from build123d import *

# Parameters (mm, degrees)
EXTRUSION1_DEPTH = 182
CONG_1_R         = 0.5


with BuildPart() as part:
    # Esquisse1 → Extrusion1 (new body)
    with BuildSketch(Plane(origin=(0, 0, 0), x_dir=(1, 0, 0), z_dir=(0, 1, 0))):
        with BuildLine():
            Line((5.5, 0), (-5.5, 0))
            Line((-5.5, 0), (-5.5, 2.476845379))
            ThreePointArc((-5.5, 2.476845379), (-4.1, 4), (-5.5, 5.523154621))
            Line((-5.5, 5.523154621), (-5.5, 6))
            Line((-5.5, 6), (-4.9, 6))
            ThreePointArc((-4.9, 6), (-3.5, 4), (-4.9, 2))
            Line((-4.9, 2), (-4.9, 0.6))
            Line((-4.9, 0.6), (4.9, 0.6))
            Line((4.9, 0.6), (4.9, 2))
            ThreePointArc((4.9, 2), (3.5, 4), (4.9, 6))
            Line((4.9, 6), (5.5, 6))
            Line((5.5, 6), (5.5, 5.523154621))
            ThreePointArc((5.5, 5.523154621), (4.1, 4), (5.5, 2.476845379))
            Line((5.5, 2.476845379), (5.5, 0))
        make_face()
    extrude(amount=EXTRUSION1_DEPTH)

    # Congé1
    cong_1_edges = [part.edges().sort_by_distance(p)[0] for p in [
        (5.5, 91, 0),
        (-5.5, 91, 0),
    ]]
    fillet(cong_1_edges, radius=CONG_1_R)


solid = part.part
Source: CAD feature listing. Evaluate the final solid. Frame: model axes, mm. A direction names the side the tool comes from. Coordinates: 2 decimals unless noted, no trailing zeros. Order: outer loops, then holes, each group sorted by start corner. A loop starts at its lowest first (then second) coordinate and runs counter-clockwise, first axis right, second up. Notation, with made-up numbers: M 37.5,-3 L 58.5,-3 A15 cw 58.5,7 Z; hole C -8.5,22 d2. An arc over 180 degrees is marked long. Write each question's results on one line, items separated by ' | '. Start each with the question number.
1. Section B-B, the plane z = -4.5. Return the cut outline in (x, y), then the cut area to 3 significant figures.
2. Section A-A, the plane y = 146. Return the cut outline in (x, z), then the cut area to 3 significant figures.
3. Pin query (flat end, axial travel): pin 1 (3 mm diameter, centred on x = 4, z = -2.5, fed in from -Y); pin 2 (5 mm diameter, centred on x = 0, y = 125, fed in from -Z). Return the tip coordinate at first contact, or that it passes through.
4. Draft query along Z for faces 3 (the face through (0, 90, 0)), 4 (the face through (0, 90, -0.6)), 5 (the face through (0, 182, -0.3)). Return one class per face: +Z half, -Z half, draft (parallel to the pull), parting line (faces both ways), or undercut.
5. Section C-C, the plane x = 0.75. Return the cut outline in (y, z), then the cut area to 3 significant figures.
6. Material intervals for L1, parallel to X at y = 138, z = -1.5; L2, parallel to Z at x = 4.25, y = 138; L3, parallel to X at y = 52, z = -3.9, sorted ascending.
7. Reachability of faces 1 (the face through (-4.1, 89.7, -4)), 2 (the face through (-3.5, 89.7, -4)) from +Z, -Z, +X, -X, +Y, -Y: full face, straight path, thin tool, end or side. Return the list, or none.
Solution:
1) outline: M -4.18,0 L -3.56,0 L -3.56,182 L -4.18,182 Z; M 3.56,0 L 4.18,0 L 4.18,182 L 3.56,182 Z | area: 227 mm²
2) outline: M -5.5,-6 L -4.9,-6 A2.13 ccw -4.9,-2 L -4.9,-0.6 L 4.9,-0.6 L 4.9,-2 A2.13 ccw 4.9,-6 L 5.5,-6 L 5.5,-5.52 A1.53 cw 5.5,-2.48 L 5.5,-0.5 A0.5 ccw 5,0 L -5,0 A0.5 ccw -5.5,-0.5 L -5.5,-2.48 A1.53 cw -5.5,-5.52 Z | area: 14.6 mm²
3) pin 1: y = 0 | pin 2: z = -0.6
4) face 3: +Z half | face 4: undercut | face 5: draft
5) outline: M 0,-0.6 L 182,-0.6 L 182,0 L 0,0 Z | area: 109 mm²
6) L1: -5.5 to -4.9, 4.9 to 5.5 | L2: -5.62 to -4.66, -3.34 to -2.38, -0.6 to 0 | L3: -4.1 to -3.5, 3.5 to 4.1
7) face 1: -X, +Y, -Y | face 2: +Y, -Y
